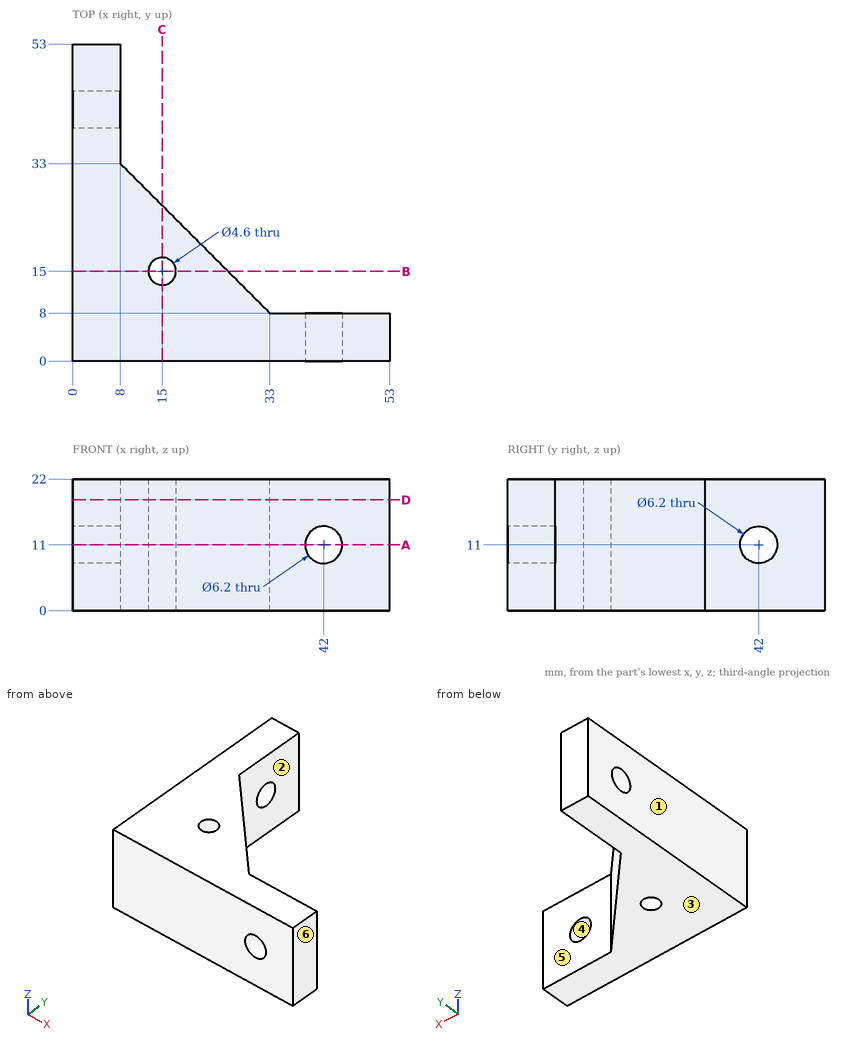
The figure shows three views and two pictorial views of one solid part (mm, origin at its lowest corner). Answer the questions. A direction names the side the tool comes from. Give positions to 0.01 mm unless a question says otherwise; leave off trailing zeros. Write each loop counter-clockwise with the first axis right and the second up, starting at its lowest first coordinate (ties: lowest second). Pieces come first, ordered by that corner, then holes. Notation, with made-up numbers: (87, 3) -> (135, 3) arc R18 cw to (135, 32) -> close; hole circle Ø5 at (12, 27). An arc over 180 degrees is marked (long way). Use one line per item in the form item = value.
1) Each of these flat-tipped pins is pushed along its axis until it touches: P1, Ø1, axis at x = 46, z = 17.5, coming from the -Y side; P2, Ø1, axis at x = 39.5, z = 4, coming from the +Y side; P3, Ø3, axis at x = 19.5, z = 6.5, coming from the +Y side; P4, Ø3, axis at y = 37.5, z = 12.5, coming from the +X side. Where does it stop, or does it pass through?
Result:
P1 = 0
P2 = 8
P3 = 23
P4 = 8
2) Straight lines are drawn through the part: probe 1 along Y at (x, z) = (4.5, 11); probe 2 along Z at (x, y) = (42, 6.25). For each, find the intervals that lie inside material, in ascending order.
Result:
probe_1 = 0 to 38.9, 45.1 to 53
probe_2 = 0 to 7.9, 14.1 to 22
3) Section B-B on y = 15 is taken. Write down the section's boundary in (x, z), plus the area to 3 significant figures.
Result:
outline = (0, 0) -> (12.7, 0) -> (12.7, 22) -> (0, 22) -> close; (17.3, 0) -> (26, 0) -> (26, 22) -> (17.3, 22) -> close
area = 471 mm²
4) Section D-D on z = 18.5 is taken. Write down the section's boundary in (x, y).
Result:
outline = (0, 0) -> (53, 0) -> (53, 8) -> (33, 8) -> (8, 33) -> (8, 53) -> (0, 53) -> close; hole circle Ø4.6 at (15, 15)
5) Section A-A on z = 11 is taken. Write down the section's boundary in (x, y).
Result:
outline = (0, 0) -> (38.9, 0) -> (38.9, 8) -> (33, 8) -> (8, 33) -> (8, 38.9) -> (0, 38.9) -> close; (0, 45.1) -> (8, 45.1) -> (8, 53) -> (0, 53) -> close; (45.1, 0) -> (53, 0) -> (53, 8) -> (45.1, 8) -> close; hole circle Ø4.6 at (15, 15)
6) For a pull along X with two mould halves and no side action, classify the marked faces 1, 2, 3 and 4 as +X half, -X half, draft (parallel to the pull), parting line (faces both ways), or undercut.
Result:
face_1 = -X half
face_2 = +X half
face_3 = draft
face_4 = undercut
7) A tool of negligible diameter and unlimited length cuts with its end or side. For the marked faces 5 and 6, from which of +Z, -Z, +X, -X, +Y, -Y can it reach the whole face along a straight path? Write none if from no direction.
Result:
face_5 = +Z, -Z, +X, +Y
face_6 = +Z, -Z, +X, +Y, -Y
